```python
from build123d import *

# Parameters (mm, degrees)
SKETCH1_W            = 63.5
SKETCH1_H            = 63.5
BOSS_EXTRUDE1_DEPTH  = 2.54
SKETCH2_R            = 1.5
CUT_EXTRUDE1_DEPTH   = 2.54
LPATTERN1_COUNT      = 2
LPATTERN1_PITCH      = 50.8
LPATTERN1_COUNT_DIR2 = 2
LPATTERN1_PITCH_DIR2 = 50.8


with BuildPart() as part:
    # Sketch1 → Boss-Extrude1 (new body)
    with BuildSketch(Plane.XY):
        with Locations((31.75, 31.75)):
            Rectangle(SKETCH1_W, SKETCH1_H)
    extrude(amount=BOSS_EXTRUDE1_DEPTH)

    # Sketch2 → Cut-Extrude1 (cut)
    with BuildSketch(Plane.XY.offset(2.54)):
        with Locations((6.35, 57.15)):
            Circle(SKETCH2_R)
    cut_extrude1 = extrude(amount=-CUT_EXTRUDE1_DEPTH, mode=Mode.SUBTRACT)

    # LPattern1: Cut-Extrude1 2 × 2
    with Locations(*[(i * LPATTERN1_PITCH, -j * LPATTERN1_PITCH_DIR2, 0) for i in range(LPATTERN1_COUNT) for j in range(LPATTERN1_COUNT_DIR2) if (i, j) != (0, 0)]):
        add(cut_extrude1, mode=Mode.SUBTRACT)


solid = part.part
```
CAD build for the part. Positions are in the model's coordinates, mm. Give positions to 0.01 mm unless a question says otherwise; leave off trailing zeros. Order: outer loops, then holes, each group sorted by start corner. A loop starts at its lowest first (then second) coordinate and runs counter-clockwise, first axis right, second up.
(1) Drill centre line: L1, parallel to Y at x = 57.15, z = 1.45. Where is it in solid material? Low to high.
(2) Flat gauge pin, fed straight in: pin 1 (4 mm diameter, centred on x = 6.35, y = 57.15, fed in from -Z). Where does the tip first touch, or does it go through?
(3) Saw through at A-A, the plane x = 6.35. Give the cut face in (y, z).
Results found:
1. L1: y = 0 to 4.85, 7.85 to 55.65, 58.65 to 63.5
2. pin 1: stops at z = 0
3. outline: (0, 0) - (4.85, 0) - (4.85, 2.54) - (0, 2.54) - close; (7.85, 0) - (55.65, 0) - (55.65, 2.54) - (7.85, 2.54) - close; (58.65, 0) - (63.5, 0) - (63.5, 2.54) - (58.65, 2.54) - close
